The listing builds one solid part. Answer for the finished solid, in the listing's coordinates (mm). A direction names the side the tool comes from. Round coordinates to 2 decimals unless told otherwise and drop trailing zeros. Loops run counter-clockwise (first coordinate to the right, second up) from the corner with the lowest first, then second, coordinate; pieces in that order, holes last. Notation, with made-up numbers: (14.25, 63) -> (31.25, 63) arc R28 cw to (31.25, 86) -> close; hole circle Ø8 at (71.5, 51.5). An arc over 180 degrees is marked (long way). Answer in a Markdown table with one row per item. Add a question column.
```python
from build123d import *

# Parameters (mm, degrees)
F0_W     = 406.4
F0_H     = 203.2
F1_DEPTH = 76.2
F2_W     = 406.4
F2_H     = 50.8
F3_DEPTH = 101.6
F5_DEPTH = 38.1


with BuildPart() as f1:
    # F0 (on Front) → F1 (new body)
    with BuildSketch(Plane.XZ):
        with Locations((-124.183113, 14.692131)):
            Rectangle(F0_W, F0_H)
    extrude(amount=F1_DEPTH)

    # F2 (on face) → F3 (join)
    with BuildSketch(Plane.XZ.offset(76.2)):
        with Locations((-124.183113, 14.692131)):
            Rectangle(F2_W, F2_H)
    extrude(amount=F3_DEPTH)

    # F4 (on face) → F5 (join, symmetric)
    with BuildSketch(Plane(origin=(0, 0, -10.707869), x_dir=(1, 0, 0), z_dir=(0, 0, -1))):
        Polygon((-406.123113, 741.68), (-406.123113, 177.8), (-327.383113, 177.8), (79.016887, 177.8), (157.756887, 177.8), (157.756887, 741.68), align=None)
    extrude(amount=F5_DEPTH, both=True)


solid = f1.part
```
Item 1: For faces 5 (the flat face through (79.017, -68, 13)), 6 (the flat face through (-128, -464, -48.808)), 7 (the flat face through (-127, -38, -86.908)), 8 (the flat face through (-127, -126, 40.092)), 9 (the flat face through (-127, -126, -10.708)), determine the directions among +Z, -Z, +X, -X, +Y, -Y from which every point of the face is accessible in a straight line to the end or side of a thin tool.
Item 2: Consider L1, parallel to Y at x = -194.5, z = -29.5; L2, parallel to Z at x = -31, y = -556.5; L3, parallel to Y at x = -94, z = 43.5. Determine where each line is inside the solid, lowest interval first. Write a range as from..to.
Item 3: Section A-A, the plane x = -226 is taken. Write down the section's boundary in (y, z).
Item 4: The mould has two halves that part along Y. Classify faces 1 (the flat face through (-127, -76.2, -48)), 2 (the flat face through (-120, -741.68, -11)), 3 (the flat face through (-327.383, -68, 13)), 4 (the flat face through (-128, -177.8, -20)): +Y half, -Y half, draft (parallel to the pull), parting line (faces both ways), or undercut.
Item 5: Section C-C, the plane y = -111 is taken. Write down the section's boundary in (x, z), and give its area (3 significant figures).
Item 6: Section B-B, the plane z = -71.5 is taken. Write down the section's boundary in (x, y).
Item 7: Flat-ended cylindrical pins translate along their axes: P1, Ø1.5, axis at x = -39.5, z = 32.5, coming from the -Y side; P2, Ø4, axis at x = -72.5, z = 58, coming from the -Y side; P3, Ø5, axis at x = -227.5, y = -163.5, coming from the -Z side. Find the tip coordinate at first contact, or state that the pin passes through.
Here are the results:
| question | item | result |
|---|---|---|
| 1 | face 5 | +Z, -Z, +X, +Y |
| 1 | face 6 | -Z, +X, -X, -Y |
| 1 | face 7 | -Z, +X, -X, +Y, -Y |
| 1 | face 8 | +Z, +X, -X, -Y |
| 1 | face 9 | -Z, +X, -X |
| 2 | L1 | y = -741.68..-177.8, -76.2..0 |
| 2 | L2 | z = -48.81..27.39 |
| 2 | L3 | y = -76.2..0 |
| 3 | outline | (-741.68, -48.81) -> (-177.8, -48.81) -> (-177.8, -10.71) -> (-76.2, -10.71) -> (-76.2, -86.91) -> (0, -86.91) -> (0, 116.29) -> (-76.2, 116.29) -> (-76.2, 40.09) -> (-177.8, 40.09) -> (-177.8, 27.39) -> (-741.68, 27.39) -> close |
| 4 | face 1 | undercut |
| 4 | face 2 | -Y half |
| 4 | face 3 | draft |
| 4 | face 4 | undercut |
| 5 | outline | (-327.38, -10.71) -> (79.02, -10.71) -> (79.02, 40.09) -> (-327.38, 40.09) -> close |
| 5 | area | 20,600 mm² |
| 6 | outline | (-327.38, -76.2) -> (79.02, -76.2) -> (79.02, 0) -> (-327.38, 0) -> close |
| 7 | P1 | stops at y = -177.8 |
| 7 | P2 | stops at y = -76.2 |
| 7 | P3 | stops at z = -10.71 |
